from build123d import *

# Parameters (mm, degrees)
EXTRUDE_1_DEPTH = 3


with BuildPart() as part:
    # 草图2 → 凸台-拉伸1 (new body)
    with BuildSketch(Plane(origin=(0, 0, 0), x_dir=(1, 0, 0), z_dir=(0, 1, 0))):
        Polygon((15, -7.5), (15, 7.5), (25, 12.5), (25, 21.65), (20, 21.65), (20, 24.65), (10, 24.65), (10, 21.65), (-10, 21.65), (-10, 24.65), (-20, 24.65), (-20, 21.65), (-25, 21.65), (-25, 12.5), (-15, 7.5), (-15, -7.5), (-25, -12.5), (-25, -21.65), (-20, -21.65), (-20, -24.65), (-10, -24.65), (-10, -21.65), (10, -21.65), (10, -24.65), (20, -24.65), (20, -21.65), (25, -21.65), (25, -12.5), align=None)
        with BuildLine():
            Line((-2.5, 7.5), (-2.5, -7.5))
            ThreePointArc((-2.5, -7.5), (0, -10), (2.5, -7.5))
            Line((2.5, -7.5), (2.5, 7.5))
            ThreePointArc((2.5, 7.5), (0, 10), (-2.5, 7.5))
        make_face(mode=Mode.SUBTRACT)
    extrude(amount=EXTRUDE_1_DEPTH)


solid = part.part
Design review of the part built by this model. Coordinates are the model's own, in mm. A direction names the side the tool comes from. Coordinates: 2 decimals unless noted, no trailing zeros. Loops run counter-clockwise (first coordinate to the right, second up) from the corner with the lowest first, then second, coordinate; pieces in that order, holes last. Notation, with made-up numbers: (0, 3.25) -> (39, 3.25) arc R9 cw to (39, 16.25) -> close; hole circle Ø8 at (76.25, -25). An arc over 180 degrees is marked (long way). Use a Markdown table: item, result. Add a question column.
Item 1: Wall thickness on L1, parallel to X at y = 0.85, z = -1; L2, parallel to Z at x = 4, y = 0.6; L3, parallel to Z at x = 20.5, y = 1.25: over which ranges is each line inside the solid? List them lowest first. Write a range as from..to.
Item 2: Machinability: for faces 1 (the flat face through (-22, 1, -21.65)), 2 (the flat face through (-15, 1, 0)), 3 (the flat face through (10, 1, 23)), 4 (the flat face through (-23, 1, 21.65)), which of the approach directions +Z, -Z, +X, -X, +Y, -Y give a long, thin tool a straight path to every point of the face, cutting with its end or side? Answer none if there is none.
Item 3: We need section D-D, the plane x = 7. Write out the cut boundary in (y, z), and give its area (3 significant figures).
Item 4: We need section C-C, the plane z = -9. Write out the cut boundary in (x, y).
Item 5: Clearance check with flat-ended pins moving along their axes: P1, Ø0.9, axis at y = 2, z = -2, coming from the -X side; P2, Ø1, axis at x = -9.5, z = -17.5, coming from the -Y side; P3, Ø1.5, axis at y = 1, z = 23, coming from the -X side; P4, Ø1.5, axis at y = 2, z = -23.5, coming from the +X side. State where each tip first meets the part, or that it passes through.
Item 6: We need section A-A, the plane x = 0. Write out the cut boundary in (y, z), and give its area (3 significant figures).
Numbers:
| question | item | result |
|---|---|---|
| 1 | L1 | x = -15..-2.5, 2.5..15 |
| 1 | L2 | z = -21.65..21.65 |
| 1 | L3 | z = -21.65..-10.25, 10.25..21.65 |
| 2 | face 1 | -Z, -X, +Y, -Y |
| 2 | face 2 | -X, +Y, -Y |
| 2 | face 3 | +Z, +Y, -Y |
| 2 | face 4 | +Z, -X, +Y, -Y |
| 3 | outline | (0, -21.65) -> (3, -21.65) -> (3, 21.65) -> (0, 21.65) -> close |
| 3 | area | 130 mm^2 |
| 4 | outline | (-18, 0) -> (-2, 0) -> (-2, 3) -> (-18, 3) -> close; (2, 0) -> (18, 0) -> (18, 3) -> (2, 3) -> close |
| 5 | P1 | stops at x = -15 |
| 5 | P2 | stops at y = 0 |
| 5 | P3 | stops at x = -20 |
| 5 | P4 | stops at x = 20 |
| 6 | outline | (0, -21.65) -> (3, -21.65) -> (3, -10) -> (0, -10) -> close; (0, 10) -> (3, 10) -> (3, 21.65) -> (0, 21.65) -> close |
| 6 | area | 69.9 mm^2 |
